```python
from build123d import *

# Parameters (mm, degrees)
F1_DEPTH = 4
F3_DEPTH = 6
F5_DEPTH = 2
F7_DEPTH = 7
F8_R     = 1.5
F9_DEPTH = 10.001


with BuildPart() as f1:
    # F0 (on Front) → F1 (new body)
    with BuildSketch(Plane.XZ):
        with BuildLine():
            ThreePointArc((20.263158, 2.446095), (11, -0.508067), (1.736842, 2.446095))
            ThreePointArc((1.736842, 2.446095), (-2.082163, 2.159767), (-2.507986, -1.64621))
            ThreePointArc((-2.507986, -1.64621), (0.593406, -15.288544), (-6.004354, -27.62554))
            ThreePointArc((-6.004354, -27.62554), (-6.26024, -30.354478), (-3.551962, -30.776156))
            ThreePointArc((-3.551962, -30.776156), (11.985415, -17.624993), (24.537749, -1.599947))
            ThreePointArc((24.537749, -1.599947), (24.062275, 2.178767), (20.263158, 2.446095))
        make_face()
    extrude(amount=F1_DEPTH)

    # F2 (on face) → F3 (join)
    with BuildSketch(Plane.XZ.offset(4)):
        with BuildLine():
            ThreePointArc((7.754053, -1.968417), (5.68946, -5.624059), (2.057931, -7.730777))
            ThreePointArc((2.057931, -7.730777), (0.908195, -8.554249), (0.590568, -9.932333))
            ThreePointArc((0.590568, -9.932333), (-0.487406, -19.606222), (-6.004354, -27.62554))
            ThreePointArc((-6.004354, -27.62554), (-6.26024, -30.354478), (-3.551962, -30.776156))
            ThreePointArc((-3.551962, -30.776156), (8.352605, -21.210498), (18.661792, -9.94368))
            ThreePointArc((18.661792, -9.94368), (19.049057, -8.320033), (18.069983, -6.968139))
            ThreePointArc((18.069983, -6.968139), (15.645578, -4.860177), (14.245947, -1.968417))
            ThreePointArc((14.245947, -1.968417), (13.477217, -0.838298), (12.162164, -0.465804))
            ThreePointArc((12.162164, -0.465804), (11, -0.508067), (9.837836, -0.465804))
            ThreePointArc((9.837836, -0.465804), (8.522783, -0.838298), (7.754053, -1.968417))
        make_face()
    extrude(amount=F3_DEPTH)

    # F4 (on face) → F5 (cut)
    with BuildSketch(Plane.XZ.offset(10)):
        with BuildLine():
            ThreePointArc((1.581491, -9.797902), (0.449618, -19.955486), (-5.343177, -28.37577))
            ThreePointArc((-5.343177, -28.37577), (-5.47112, -29.740239), (-4.116981, -29.951078))
            ThreePointArc((-4.116981, -29.951078), (7.66854, -20.481077), (17.874636, -9.326927))
            ThreePointArc((17.874636, -9.326927), (18.068268, -8.515104), (17.578731, -7.839157))
            ThreePointArc((17.578731, -7.839157), (14.851275, -5.467699), (13.276691, -2.214469))
            ThreePointArc((13.276691, -2.214469), (12.892325, -1.649409), (12.234799, -1.463162))
            ThreePointArc((12.234799, -1.463162), (11, -1.508067), (9.765201, -1.463162))
            ThreePointArc((9.765201, -1.463162), (9.107675, -1.649409), (8.723309, -2.214469))
            ThreePointArc((8.723309, -2.214469), (6.400643, -6.327067), (2.315173, -8.697125))
            ThreePointArc((2.315173, -8.697125), (1.740304, -9.108861), (1.581491, -9.797902))
        make_face()
    extrude(amount=-F5_DEPTH, mode=Mode.SUBTRACT)

    # F6 (on face) → F7 (cut)
    with BuildSketch(Plane.XZ.offset(8)):
        with BuildLine():
            ThreePointArc((-4.682, -29.126), (6.984475, -19.751655), (17.087479, -8.710174))
            ThreePointArc((17.087479, -8.710174), (14.056973, -6.075221), (12.307434, -2.460521))
            ThreePointArc((12.307434, -2.460521), (11, -2.508067), (9.692566, -2.460521))
            ThreePointArc((9.692566, -2.460521), (7.111825, -7.030074), (2.572414, -9.663472))
            ThreePointArc((2.572414, -9.663472), (1.386642, -20.30475), (-4.682, -29.126))
        make_face()
    extrude(amount=-F7_DEPTH, mode=Mode.SUBTRACT)

    # F8 (on Front) → F9 (cut, through all)
    with BuildSketch(Plane.XZ):
        Circle(F8_R)
        with Locations((22, 0)):
            Circle(F8_R)
    extrude(amount=F9_DEPTH, mode=Mode.SUBTRACT)

    # F10: F1 across face


with BuildPart() as f1_1:
    add(f1.part)
    add(f1.part.mirror(Plane(origin=(5.783176, -10, -15.645769), x_dir=(1, 0, 0), z_dir=(0, -1, 0))))


solid = f1_1.part
```
CAD build for the part. Positions are in the model's coordinates, mm. A direction names the side the tool comes from. Coordinates: 2 decimals unless noted, no trailing zeros. Order: outer loops, then holes, each group sorted by start corner. A loop starts at its lowest first (then second) coordinate and runs counter-clockwise, first axis right, second up. Notation, with made-up numbers: (27, 87.5) - (82, 87.5) arc R25 ccw to (82, 106.5) - close; hole circle Ø7 at (77, 67.5). An arc over 180 degrees is marked (long way). Use a Markdown table: item, result. Add a question column.
(1) Saw through at A-A (z = 0). Count the separate pieces of the cut face and the enclosed holes in it, then the cut area to 3 significant figures.
(2) Drill centre lines: line 1 along Z through (x, y) = (22, -18.4); line 2 along X through (y, z) = (-17.25, -28.5); line 3 along Y through (x, z) = (23, -2). Where is each one in solid material? Low to high. Write a range as [from, to].
(3) Which spindle directions (+Z, -Z, +X, -X, +Y, -Y) get a long thin tool onto all of the face, cutting with end or side? Do faces 1 (the face through (3, -4, -3)), 2 (the face through (19, -16, -3)), 3 (the face through (19.054, -10.084, -8.344)), 4 (the face through (6.448, -9.972, -6.279)). Say none if no direction does.
(4) Flat gauge pins, fed straight in: pin 1 (2.5 mm diameter, centred on x = 0, z = 0, fed in from +Y); pin 2 (1.5 mm diameter, centred on x = 8.5, y = -12, fed in from -Z); pin 3 (10 mm diameter, centred on y = -18, z = -16, fed in from -X); pin 4 (1 mm diameter, centred on y = -2, z = -13, fed in from -X). Where does each tip first touch, or does it go through?
(5) Pull direction Y, two halves, no side cores. Call faces 5 (the face through (1.746, -9.972, -9.1)), 6 (the face through (-1.5, -18.03, 0.07)), 7 (the face through (8.539, -10.084, -0.827)): +Y half, -Y half, draft (parallel to the pull), parting line (faces both ways), or undercut.
(6) Saw through at B-B (x = 22). Give the cut face in (y, z).
(7) Saw through at D-D (y = -1.5). Give the cut face in (x, z), then the cut area to 3 significant figures.
Solved:
| question | item | result |
|---|---|---|
| 1 | separate pieces | 8 |
| 1 | enclosed holes | 0 |
| 1 | area | 112 mm² |
| 2 | line 1 | z = [-5.43, -1.5], [1.5, 3] |
| 2 | line 2 | x = [-6.58, -4], [-3.78, -0.36] |
| 2 | line 3 | y = [-20, -16], [-4, 0] |
| 3 | face 1 | +Z, -X |
| 3 | face 2 | +Z, +X |
| 3 | face 3 | +X |
| 3 | face 4 | none |
| 4 | pin 1 | passes through |
| 4 | pin 2 | stops at z = -21.77 |
| 4 | pin 3 | stops at x = -1.07 |
| 4 | pin 4 | stops at x = 0.75 |
| 5 | face 5 | undercut |
| 5 | face 6 | draft |
| 5 | face 7 | undercut |
| 6 | outline | (-20, -5.43) - (-16, -5.43) - (-16, -1.5) - (-20, -1.5) - close; (-20, 1.5) - (-16, 1.5) - (-16, 3) - (-20, 3) - close; (-4, -5.43) - (0, -5.43) - (0, -1.5) - (-4, -1.5) - close; (-4, 1.5) - (0, 1.5) - (0, 3) - (-4, 3) - close |
| 7 | outline | (-6, -27.63) arc R2 ccw to (-3.55, -30.78) arc R100 ccw to (24.54, -1.6) arc R3 ccw to (20.26, 2.45) arc R16 cw to (1.74, 2.45) arc R3 ccw to (-2.51, -1.65) arc R20 cw to start; hole (-4.68, -29.13) arc R98 ccw to (17.09, -8.71) arc R10 cw to (12.31, -2.46) arc R18 cw to (9.69, -2.46) arc R10 cw to (2.57, -9.66) arc R22 cw to start; hole circle Ø3 at (0, 0); hole circle Ø3 at (22, 0) |
| 7 | area | 301 mm² |
